Verification items for the finished model (mm, model axes). Face numbers are marked on the shaded views. Coordinates: 2 decimals unless noted, no trailing zeros. Loops run counter-clockwise (first coordinate to the right, second up) from the corner with the lowest first, then second, coordinate; pieces in that order, holes last. Notation, with made-up numbers: (-9.5, -15.5) - (45.5, -15.5) arc R15 ccw to (45.5, 9.5) - close; hole circle Ø1 at (60.25, 51.25). An arc over 180 degrees is marked (long way). Answer as CSV lines item,"result". Start each with the question number.
1. Cross-section at A-A (x = 0). Enter the section's corners in (y, z), plus the area to 3 significant figures.
2. Material ranges on line 1 (Y direction, x = 0, z = 38.5); line 2 (Y direction, x = 2, z = 34); line 3 (X direction, y = -1, z = 35.5), recorded low to high. Write a range as [from, to].
3. Release check for a two-part mould opening along X. For the marked faces 1 and 2 record: pulls with the +X half, pulls with the -X half, needs draft (parallel to the pull), parting line crosses it, or undercut.
4. Gauge pin test, flat ends, axial feed: P1, Ø4, axis at x = 1, y = 4, coming from the -Z side; P2, Ø1, axis at x = 4.5, z = 18.5, coming from the -Y side; P3, Ø10, axis at y = 6.5, z = 37, coming from the +X side. Record the tip position at first contact, or that the pin passes through.
5. Cross-section at C-C (z = 27). Enter the section's corners in (x, y).
```python
from build123d import *

# Parameters (mm, degrees)
ESQUISSE1_R      = 9.5
EXTRUSION1_DEPTH = 50.8
ESQUISSE2_R      = 5.75
EXTRUSION2_DEPTH = 53.546550791
FILLET1_R        = 1


with BuildPart() as part:
    # Esquisse1 → Extrusion1 (new body)
    with BuildSketch(Plane.XY):
        Circle(ESQUISSE1_R)
    extrude(amount=EXTRUSION1_DEPTH)

    # Esquisse2 → Extrusion2 (cut, through all)
    with BuildSketch(Plane.XY.offset(50.8)):
        Circle(ESQUISSE2_R)
    extrude(amount=-EXTRUSION2_DEPTH, mode=Mode.SUBTRACT)

    # Fillet1
    fillet1_edges = [part.edges().sort_by_distance(p)[0] for p in [
        (-9.5, 0, 0),
        (-9.5, 0, 50.8),
        (-5.75, 0, 0),
        (-5.75, 0, 50.8),
    ]]
    fillet(fillet1_edges, radius=FILLET1_R)


solid = part.part
```
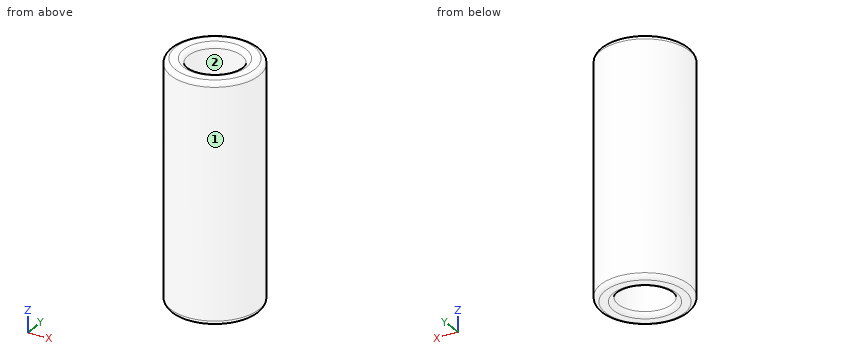
Values follow:
1,outline,"(-9.5, 1) arc R1 ccw to (-8.5, 0) - (-6.75, 0) arc R1 ccw to (-5.75, 1) - (-5.75, 49.8) arc R1 ccw to (-6.75, 50.8) - (-8.5, 50.8) arc R1 ccw to (-9.5, 49.8) - close; (5.75, 1) arc R1 ccw to (6.75, 0) - (8.5, 0) arc R1 ccw to (9.5, 1) - (9.5, 49.8) arc R1 ccw to (8.5, 50.8) - (6.75, 50.8) arc R1 ccw to (5.75, 49.8) - close"
1,area,"379 mm²"
2,line 1,"y = [-9.5, -5.75], [5.75, 9.5]"
2,line 2,"y = [-9.29, -5.39], [5.39, 9.29]"
2,line 3,"x = [-9.45, -5.66], [5.66, 9.45]"
3,face 1,"parting line crosses it"
3,face 2,"undercut"
4,P1,"stops at z = 0.22"
4,P2,"stops at y = -8.62"
4,P3,"stops at x = 9.38"
5,outline,"circle Ø19 at (0, 0); hole circle Ø11.5 at (0, 0)"
